Job drawing, mm, ordinate dimensions from the low corner. One solid piece. A direction names the side the tool comes from. Give positions to 0.01 mm unless a question says otherwise; leave off trailing zeros. Order: outer loops, then holes, each group sorted by start corner. A loop starts at its lowest first (then second) coordinate and runs counter-clockwise, first axis right, second up. Notation, with made-up numbers: M 20.25,50.25 L 33.25,50.25 A6 ccw 33.25,54.25 Z; hole C 37.5,75 d8. An arc over 180 degrees is marked long. One line per item, written item: value. Start each with the question number.
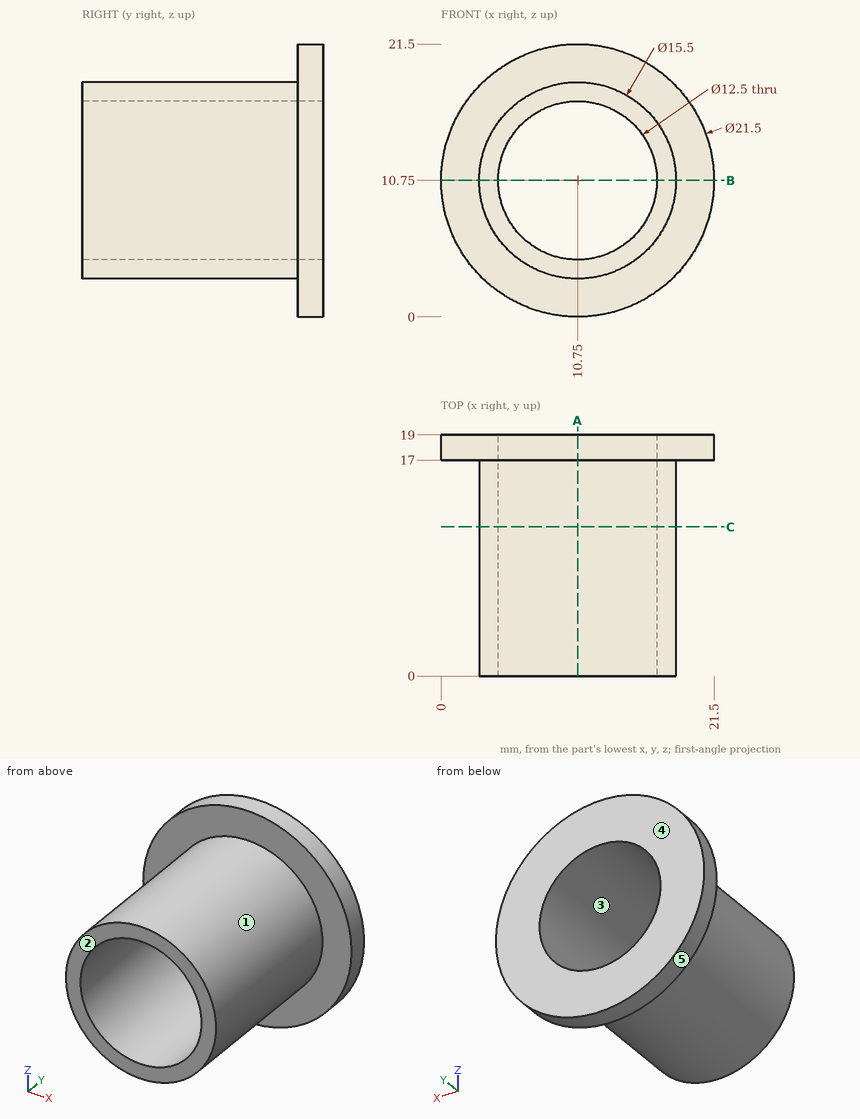
1) Drill centre lines: line 1 (Z direction, x = 10.75, y = 4.5); line 2 (X direction, y = 11.75, z = 11) (3 decimals); line 3 (Y direction, x = 8.75, z = 19.25). Where is each one in solid material? Low to high.
2) Slice it at C-C (y = 11.75). List the corners of the cut face in (x, z), plus the area to 3 significant figures.
3) Slice it at B-B (z = 10.75). List the corners of the cut face in (x, y), plus the area to 3 significant figures.
4) Slice it at A-A (x = 10.75). List the corners of the cut face in (y, z).
5) Pull direction X, two halves, no side cores. Call the marked faces 3, 4 and 5: pulls with the +X half, pulls with the -X half, needs draft (parallel to the pull), parting line crosses it, or undercut.
6) Tool access for the marked faces 1 and 2: list every direction of +Z, -Z, +X, -X, +Y, -Y with a clear straight run to the whole face (end or side of a thin tool).
7) Drop flat-ended pins along their axis: P1, Ø4, axis at y = 8.5, z = 5.5, coming from the +X side; P2, Ø1.5, axis at y = 16, z = 7.5, coming from the -X side; P3, Ø10, axis at x = 4, y = 16.5, coming from the -Z side. Give the stop position or say it passes through.
Results list:
1. line 1: z = 3 to 4.5, 17 to 18.5
1. line 2: x = 3.004 to 4.505, 16.995 to 18.496
1. line 3: y = 17 to 19
2. outline: C 10.75,10.75 d15.5; hole C 10.75,10.75 d12.5
2. area: 66.0 mm²
3. outline: M 0,17 L 3,17 L 3,0 L 4.5,0 L 4.5,19 L 0,19 Z; M 17,0 L 18.5,0 L 18.5,17 L 21.5,17 L 21.5,19 L 17,19 Z
3. area: 69.0 mm²
4. outline: M 0,3 L 17,3 L 17,0 L 19,0 L 19,4.5 L 0,4.5 Z; M 0,17 L 19,17 L 19,21.5 L 17,21.5 L 17,18.5 L 0,18.5 Z
5. face 3: undercut
5. face 4: needs draft
5. face 5: parting line crosses it
6. face 1: -Y
6. face 2: +Z, -Z, +X, -X, -Y
7. P1: stops at x = 17.79
7. P2: stops at x = 3.41
7. P3: stops at z = 0.15
